Geometry: final body of the model. Coordinates: model frame, mm. Give positions to 0.01 mm unless a question says otherwise; leave off trailing zeros. Loops run counter-clockwise (first coordinate to the right, second up) from the corner with the lowest first, then second, coordinate; pieces in that order, holes last. Notation, with made-up numbers: (65, -27) -> (91, -27) arc R6 ccw to (91, -22) -> close; hole circle Ø3 at (58.5, 73). An arc over 180 degrees is marked (long way). Answer in a Markdown table with one row per item. Add a question column.
1) Section query A-A (y = 0). Return the cut outline in (x, z), plus the area to 3 significant figures.
2) Section query C-C (z = -112.5). Return the cut outline in (x, y), plus the area to 3 significant figures.
3) Line query: line 1 (Y direction, x = 0.5, z = -121.92); line 2 (Z direction, x = -3.5, y = 0); line 3 (Z direction, x = 13.5, y = -1.5). Output: solid intervals per line, ascending. Write a range as from..to.
4) First-contact query: P1, Ø10, axis at y = 12, z = -49.5, coming from the -X side; P2, Ø6, axis at y = 0, z = -121.92, coming from the +X side; P3, Ø2, axis at y = 10.5, z = 29, coming from the -X side; P4, Ø1.1, axis at x = 1, y = 14, coming from the +Z side. Flat tips, straight axial feed; report the tip coordinate or a pass-through.
5) Draft query along Y for faces 1 (the flat face through (0, -1, 134.62)), 2 (the cylindrical face through (-0.213, -0.496, -125.698)), 3 (the cylindrical face through (8.19, -12.85, -1.87)), 4 (the flat face through (0, 11.43, 122)). Return one class per face: +Y half, -Y half, draft (parallel to the pull), parting line (faces both ways), or undercut.
6) Section query B-B (x = 0). Return the cut outline in (y, z), plus the area to 3 significant figures.
Autodesk Inventor part; units mm, degrees
ref_plane "YZ Plane" through (0, 0, 0) normal (1, 0, 0) x (0, 1, 0)
ref_plane "XZ Plane" through (0, 0, 0) normal (0, 1, 0) x (-1, 0, 0)
ref_plane "XY Plane" through (0, 0, 0) normal (0, 0, 1) x (1, 0, 0)
sketch "Sketch1" plane through (0, 0, 0) normal (0, 0, 1) x (1, 0, 0)
  circle A0 centre (0, 0) radius 15.24
  dimension "d0" = 30.48
extrude "Extrusion1" add sketch "Sketch1" along normal mid plane 269.24
sketch "Sketch2" plane through (0, 0, 0) normal (1, 0, 0) x (0, 1, 0)
  line L0 (15.24, -134.62) -> (-15.24, -134.62)
  line L1 (-15.24, -134.62) -> (-15.24, 134.62)
  line L2 (-15.24, 134.62) -> (15.24, 134.62)
  line L3 (15.24, 134.62) -> (15.24, -134.62)
  line L4 (-15.24, -134.62) -> (15.24, -134.62)
  line L5 (15.24, 134.62) -> (-15.24, 134.62)
  circle A0 centre (0, -121.92) radius 3.81
  line L6 (19.558, 134.62) -> (11.43, 134.62)
  line L7 (11.43, 134.62) -> (11.43, 109.22)
  line L8 (11.43, 109.22) -> (19.558, 109.22)
  line L9 (19.558, 109.22) -> (19.558, 134.62)
  line L10 (0, -188.468) -> (0, 188.468)
  point P0 (0, 0)
  dimension "d3" = 7.62
  dimension "d4" = 12.7
  dimension "d5" = 8.128
  dimension "d6" = 25.4
  dimension "d7" = 11.43
extrude "Extrusion2" cut sketch "Sketch2" against normal through all both and the other way through all contours L8 L7 L2 L3 | L3 L6 L9 L8 | L10 A0 | A0 L10
chamfer "Chamfer1" distance 1.27 angle 45 3 edges at (13.8903, 6.2703, 134.62) (-6.2703, -13.8903, 134.62) (-15.24, 0, -134.62) measured on face at (-13.538, 6.9987, 44.8733)
equation "\"BendRadius\" = Thickness"
equation "\"BendReliefWidth\" = Thickness"
equation "\"BendReliefDepth\" = 0.5 * Thickness"
equation "\"CornerReliefSize\" = 4 * Thickness"
equation "\"MinimumRemnant\" = 2 * Thickness"
equation "\"TransitionRadius\" = BendRadius"
equation "\"JacobiRadiusSize\" = BendRadius"
equation "\"GapSize\" = Thickness"
properties part number "crankshaft" material "Stainless Steel"
Evaluation:
| question | item | result |
|---|---|---|
| 1 | outline | (-15.24, -133.35) -> (-13.97, -134.62) -> (13.97, -134.62) -> (15.24, -133.35) -> (15.24, -125.73) -> (-15.24, -125.73) -> close; (-15.24, -118.11) -> (15.24, -118.11) -> (15.24, 133.35) -> (13.97, 134.62) -> (-13.97, 134.62) -> (-15.24, 133.35) -> close |
| 1 | area | 7,970 mm² |
| 2 | outline | circle Ø30.48 at (0, 0) |
| 2 | area | 730 mm² |
| 3 | line 1 | -15.23..-3.81, 3.81..15.23 |
| 3 | line 2 | -134.62..-125.73, -118.11..134.62 |
| 3 | line 3 | -134.62..-125.42, -118.42..134.62 |
| 4 | P1 | x = -13.54 |
| 4 | P2 | through |
| 4 | P3 | x = -11.92 |
| 4 | P4 | z = 109.22 |
| 5 | face 1 | draft |
| 5 | face 2 | undercut |
| 5 | face 3 | parting line |
| 5 | face 4 | +Y half |
| 6 | outline | (-15.24, -133.35) -> (-13.97, -134.62) -> (13.97, -134.62) -> (15.24, -133.35) -> (15.24, 109.22) -> (11.43, 109.22) -> (11.43, 134.62) -> (-13.97, 134.62) -> (-15.24, 133.35) -> close; hole circle Ø7.62 at (0, -121.92) |
| 6 | area | 8,060 mm² |
